Here's the drawing with two shaded views (mm, measured from the low corner). I have some questions. Coordinates: 2 decimals unless noted, no trailing zeros. Order: outer loops, then holes, each group sorted by start corner. A loop starts at its lowest first (then second) coordinate and runs counter-clockwise, first axis right, second up. Notation, with made-up numbers: M 33.5,-29 L 65.5,-29 A36 ccw 65.5,7 Z; hole C 27,0.25 d7. An arc over 180 degrees is marked long. Put each result on its own line as item: value. Start each with the question number.
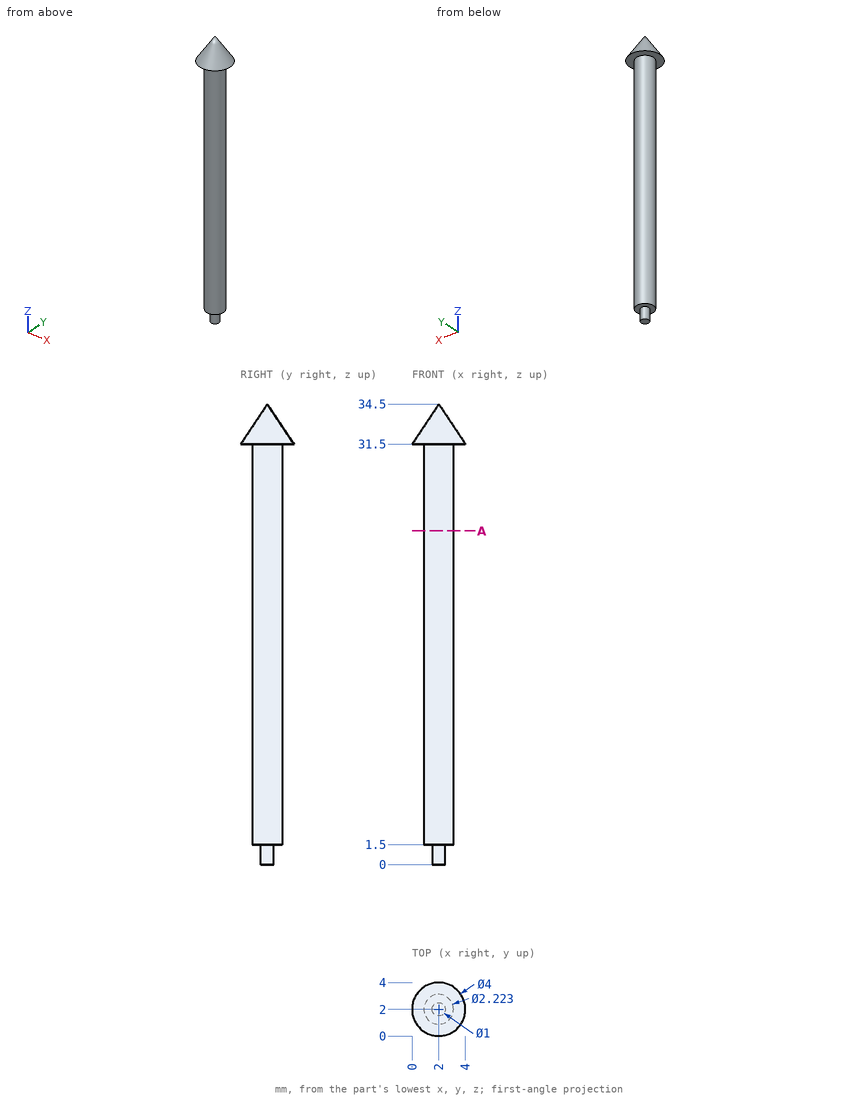
Item 1: I need wall thicknesses on probe 1 along Y at (x, z) = (1.95, 8.5); probe 2 along X at (y, z) = (2.4, 7). Which ranges of each line are inside material? Lowest first, please.
Item 2: If we section it at A-A on z = 25: Write out the boundary of the cut face in (x, y), then the cut area to 3 significant figures.
Item 3: For pin 1 Ø1.5 at (x, z) = (1.5, 14.5) entering from +Y; pin 2 Ø2 at (x, y) = (3, 0.5) entering from +Z, each with a flat end and sliding along its axis, tell me the tip position at first contact or that it passes through.
Geometry check:
1. probe 1: y = 0.89 to 3.11
1. probe 2: x = 0.96 to 3.04
2. outline: C 2,2 d2.22
2. area: 3.88 mm²
3. pin 1: stops at y = 3.11
3. pin 2: stops at z = 33.3
